Read the model definition and answer for the solid it produces. Units are mm, in the model's axes. A direction names the side the tool comes from. Give positions to 0.01 mm unless a question says otherwise; leave off trailing zeros. Write each loop counter-clockwise with the first axis right and the second up, starting at its lowest first coordinate (ties: lowest second). Pieces come first, ordered by that corner, then holes. Notation, with made-up numbers: M -15,-2.75 L 29,-2.75 A29 cw 29,33.25 Z; hole C -40,43.25 d10. An arc over 180 degrees is marked long. Use a Markdown table: item, result. Add a question column.
Item 1: Consider probe 1 along Z at (x, y) = (-76, 4.25) (3 decimals); probe 2 along X at (y, z) = (3, -11); probe 3 along Z at (x, y) = (-120.5, 1.5). Determine where each line is inside the solid, lowest interval first. Write a range as [from, to].
Item 2: A cutting plane is placed at B-B on x = 93. Determine the outline of the cut face in (y, z) (3 decimals), then the cut area to 3 significant figures.
Item 3: For faces 1 (the flat face through (-144, 5, 114.3)), 2 (the flat face through (-149.225, 5, -102)), 3 (the flat face through (144, 5, 38.1)), 4 (the flat face through (114.3, 5, -144)), 5 (the flat face through (127, 5, -149.225)), determine the directions among +Z, -Z, +X, -X, +Y, -Y from which every point of the face is accessible in a straight line to the end or side of a thin tool.
Item 4: A cutting plane is placed at A-A on z = -94.5. Determine the outline of the cut face in (x, y) (3 decimals), then the cut area to 3 significant figures.
Item 5: Given P1, Ø1, axis at y = 1, z = 106.5, coming from the -X side; P2, Ø5, axis at y = 3, z = 4.5, coming from the +X side; P3, Ø4, axis at y = 2, z = -82.5, coming from the -X side, each flat-ended and moving along its own axis, determine where each tip first touches the part or whether it passes through.
Item 6: The mould has two halves that part along X. Classify faces 6 (the flat face through (144, 5, -88.9)), 7 (the flat face through (0, 5, -139.7)), 8 (the flat face through (139.7, 5, 51)): pulls with the +X half, pulls with the -X half, needs draft (parallel to the pull), parting line crosses it, or undercut.
from build123d import *

# Parameters (mm, degrees)
SKETCH1_W               = 279.4
SKETCH1_H               = 279.4
BOSS_EXTRUDE1_DEPTH     = 9.525
SKETCH2_W               = 25.4
SKETCH2_H               = 9.525
BOSS_EXTRUDE2_DEPTH     = 9.525
LPATTERN1_COUNT         = 5
LPATTERN1_PITCH         = 50.8
MIRROR1_COPY_1_SKETCH_W = 25.4
MIRROR1_COPY_1_SKETCH_H = 9.525
MIRROR1_COPY_1_DEPTH    = 9.525
MIRROR1_COPY_2_SKETCH_W = 25.4
MIRROR1_COPY_2_SKETCH_H = 9.525
MIRROR1_COPY_2_DEPTH    = 9.525
MIRROR1_COPY_3_SKETCH_W = 25.4
MIRROR1_COPY_3_SKETCH_H = 9.525
MIRROR1_COPY_3_DEPTH    = 9.525
MIRROR1_COPY_4_SKETCH_W = 25.4
MIRROR1_COPY_4_SKETCH_H = 9.525
MIRROR1_COPY_4_DEPTH    = 9.525
SKETCH3_W               = 25.4
SKETCH3_H               = 9.525
BOSS_EXTRUDE3_DEPTH     = 9.525
LPATTERN2_COUNT         = 5
LPATTERN2_PITCH         = 50.8
SKETCH6_R               = 4.7625
CUT_EXTRUDE1_DEPTH      = 10.525
SKETCH8_W               = 84.891093183
SKETCH8_H               = 177.8
CUT_EXTRUDE3_DEPTH      = 10.525
SKETCH9_W               = 25.4
SKETCH9_H               = 9.525
BOSS_EXTRUDE4_DEPTH     = 9.525


with BuildPart() as part:
    # Sketch1 → Boss-Extrude1 (new body)
    with BuildSketch(Plane(origin=(0, 0, 0), x_dir=(1, 0, 0), z_dir=(0, 1, 0))):
        Rectangle(SKETCH1_W, SKETCH1_H)
    extrude(amount=BOSS_EXTRUDE1_DEPTH)

    # Sketch2 → Boss-Extrude2 (add)
    with BuildSketch(Plane(origin=(139.7, 0, 0), x_dir=(0, 0, -1), z_dir=(1, 0, 0))):
        with Locations((-127, 4.7625)):
            Rectangle(SKETCH2_W, SKETCH2_H)
    boss_extrude2 = extrude(amount=BOSS_EXTRUDE2_DEPTH)

    # LPattern1: Boss-Extrude2 ×5
    with Locations(*[(0, 0, -i * LPATTERN1_PITCH) for i in range(1, LPATTERN1_COUNT)]):
        add(boss_extrude2)

    # Mirror1: Boss-Extrude2 across plane
    add(boss_extrude2.mirror(Plane(origin=(0, 0, 0), x_dir=(0, 0, 1), z_dir=(1, 0, 0))))

    # Mirror1 copy 1 sketch → Mirror1 copy 1 (add)
    with BuildSketch(Plane(origin=(-139.7, 0, -50.8), x_dir=(0, 0, -1), z_dir=(-1, 0, 0))):
        with Locations((-127, -4.7625)):
            Rectangle(MIRROR1_COPY_1_SKETCH_W, MIRROR1_COPY_1_SKETCH_H)
    extrude(amount=MIRROR1_COPY_1_DEPTH)

    # Mirror1 copy 2 sketch → Mirror1 copy 2 (add)
    with BuildSketch(Plane(origin=(-139.7, 0, -101.6), x_dir=(0, 0, -1), z_dir=(-1, 0, 0))):
        with Locations((-127, -4.7625)):
            Rectangle(MIRROR1_COPY_2_SKETCH_W, MIRROR1_COPY_2_SKETCH_H)
    extrude(amount=MIRROR1_COPY_2_DEPTH)

    # Mirror1 copy 3 sketch → Mirror1 copy 3 (add)
    with BuildSketch(Plane(origin=(-139.7, 0, -152.4), x_dir=(0, 0, -1), z_dir=(-1, 0, 0))):
        with Locations((-127, -4.7625)):
            Rectangle(MIRROR1_COPY_3_SKETCH_W, MIRROR1_COPY_3_SKETCH_H)
    extrude(amount=MIRROR1_COPY_3_DEPTH)

    # Mirror1 copy 4 sketch → Mirror1 copy 4 (add)
    with BuildSketch(Plane(origin=(-139.7, 0, -203.2), x_dir=(0, 0, -1), z_dir=(-1, 0, 0))):
        with Locations((-127, -4.7625)):
            Rectangle(MIRROR1_COPY_4_SKETCH_W, MIRROR1_COPY_4_SKETCH_H)
    extrude(amount=MIRROR1_COPY_4_DEPTH)

    # Sketch3 → Boss-Extrude3 (add)
    with BuildSketch(Plane(origin=(0, 0, -139.7), x_dir=(-1, 0, 0), z_dir=(0, 0, -1))):
        with Locations((-127, 4.7625)):
            Rectangle(SKETCH3_W, SKETCH3_H)
    boss_extrude3 = extrude(amount=BOSS_EXTRUDE3_DEPTH)

    # LPattern2: Boss-Extrude3 ×5
    with Locations(*[(-i * LPATTERN2_PITCH, 0, 0) for i in range(1, LPATTERN2_COUNT)]):
        add(boss_extrude3)

    # Sketch6 → Cut-Extrude1 (cut, through all)
    with BuildSketch(Plane(origin=(0, 9.525, 0), x_dir=(1, 0, 0), z_dir=(0, 1, 0))):
        with Locations((38.1, 11.176)):
            Circle(SKETCH6_R)
    extrude(amount=-CUT_EXTRUDE1_DEPTH, mode=Mode.SUBTRACT)

    # Sketch8 → Cut-Extrude3 (cut, through all)
    with BuildSketch(Plane(origin=(0, 9.525, 0), x_dir=(1, 0, 0), z_dir=(0, 1, 0))):
        with Locations((-106.779453409, 0)):
            Rectangle(SKETCH8_W, SKETCH8_H)
    extrude(amount=-CUT_EXTRUDE3_DEPTH, mode=Mode.SUBTRACT)

    # Sketch9 → Boss-Extrude4 (add)
    with BuildSketch(Plane.ZY.offset(139.7)):
        with Locations((-101.6, 4.7625)):
            Rectangle(SKETCH9_W, SKETCH9_H)
    extrude(amount=BOSS_EXTRUDE4_DEPTH)


solid = part.part
Filled in:
| question | item | result |
|---|---|---|
| 1 | probe 1 | [-149.225, -88.9], [88.9, 139.7] |
| 1 | probe 2 | [-64.33, 33.34], [42.86, 139.7] |
| 1 | probe 3 | [-139.7, -88.9], [88.9, 139.7] |
| 2 | outline | M 0,-139.7 L 9.525,-139.7 L 9.525,139.7 L 0,139.7 Z |
| 2 | area | 2,660 mm² |
| 3 | face 1 | -X, +Y, -Y |
| 3 | face 2 | +Z, -Z, -X, +Y, -Y |
| 3 | face 3 | +X, +Y, -Y |
| 3 | face 4 | -Z, +Y, -Y |
| 3 | face 5 | -Z, +X, -X, +Y, -Y |
| 4 | outline | M -149.225,0 L 139.7,0 L 139.7,9.525 L -149.225,9.525 Z |
| 4 | area | 2,750 mm² |
| 5 | P1 | x = -139.7 |
| 5 | P2 | x = 139.7 |
| 5 | P3 | x = -64.33 |
| 6 | face 6 | needs draft |
| 6 | face 7 | undercut |
| 6 | face 8 | pulls with the +X half |
